For this review, take the finished solid that the model builds, in its own axes (mm). Face numbers are marked on the shaded views. A direction names the side the tool comes from. Give positions to 0.01 mm unless a question says otherwise; leave off trailing zeros. Loops run counter-clockwise (first coordinate to the right, second up) from the corner with the lowest first, then second, coordinate; pieces in that order, holes last. Notation, with made-up numbers: (-26, 33.5) -> (19, 33.5) arc R19 cw to (19, 70.5) -> close; hole circle Ø7 at (41.25, 26.25). An arc over 180 degrees is marked (long way). Answer as CSV lines item,"result". Start each with the question number.
Item 1: Add section A-A on y = -15.5. State the section outline as (x, z) points.
Item 2: Add section C-C on z = 7. State the section outline as (x, y) points.
Item 3: The part is to be moulded in two halves that separate along X. For the marked faces 4, 5 and 6, say which applies: +X half, -X half, draft (parallel to the pull), parting line (faces both ways), or undercut.
Item 4: For L1, parallel to Y at x = -15.5, z = 1.2; L2, parallel to Y at x = 17, z = 2.75, list the stretches that pass through material, from the lowest coordinate up. Write a range as from..to.
Item 5: Add section D-D on y = 0. State the section outline as (x, z) points, plus the area to 3 significant figures.
Item 6: Add section B-B on x = 0. State the section outline as (y, z) points, plus the area to 3 significant figures.
Item 7: Clearance check with flat-ended pins moving along their axes: P1, Ø6.5, axis at x = 16, y = 15, coming from the +Z side; P2, Ø4.5, axis at x = -17, z = 6, coming from the -Y side; P3, Ø4, axis at x = 16.5, z = 7.6, coming from the -Y side; P4, Ø23.5, axis at x = 0, y = 0, coming from the +Z side. State where each tip first meets the part, or that it passes through.
Item 8: Machinability: for the marked faces 1, 2 and 3, which of the approach directions +Z, -Z, +X, -X, +Y, -Y give a long, thin tool a straight path to every point of the face, cutting with its end or side? Answer none if there is none.
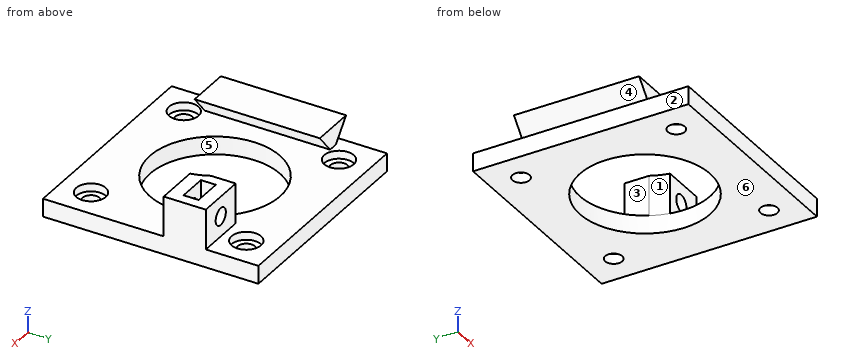
```python
from build123d import *

# Parameters (mm, degrees)
SKETCH_W        = 43
SKETCH_H        = 43
SKETCH_R        = 13
SKETCH_R_2      = 1.7
PAD_DEPTH       = 3.6
SKETCH001_R     = 2.95
POCKET_DEPTH    = 1.6
PAD001_DEPTH    = 8
SKETCH003_R     = 1.7
POCKET001_DEPTH = 18.901
POCKET002_DEPTH = 1.5
PAD002_DEPTH    = 12.5


with BuildPart() as part:
    # Sketch → Pad (new body)
    with BuildSketch(Plane.XY):
        Rectangle(SKETCH_W, SKETCH_H)
        Circle(SKETCH_R, mode=Mode.SUBTRACT)
        with Locations((-15.5, 15.5)):
            Circle(SKETCH_R_2, mode=Mode.SUBTRACT)
        with Locations((15.5, 15.5)):
            Circle(SKETCH_R_2, mode=Mode.SUBTRACT)
        with Locations((15.5, -15.5)):
            Circle(SKETCH_R_2, mode=Mode.SUBTRACT)
        with Locations((-15.5, -15.5)):
            Circle(SKETCH_R_2, mode=Mode.SUBTRACT)
    extrude(amount=PAD_DEPTH)

    # Sketch001 (on Face11 of Pad) → Pocket (cut)
    with BuildSketch(Plane.XY.offset(3.6)):
        with Locations((15.5, 15.5)):
            Circle(SKETCH001_R)
        with Locations((-15.5, 15.5)):
            Circle(SKETCH001_R)
        with Locations((-15.5, -15.5)):
            Circle(SKETCH001_R)
        with Locations((15.5, -15.5)):
            Circle(SKETCH001_R)
    extrude(amount=-POCKET_DEPTH, mode=Mode.SUBTRACT)

    # Sketch002 (on Face5 of Pocket) → Pad001 (join)
    with BuildSketch(Plane.XY.offset(3.6)):
        with BuildLine():
            ThreePointArc((12.737347, 2.6), (12.241687, 4.375053), (11.5, 6.062178))
            Line((11.5, 6.062178), (11.5, 11))
            Line((11.5, 11), (21.5, 11))
            Line((21.5, 11), (21.5, 2.6))
            Line((21.5, 2.6), (12.737347, 2.6))
        make_face()
    extrude(amount=PAD001_DEPTH)

    # Sketch003 (on Face10 of Pad001) → Pocket001 (cut, through all)
    with BuildSketch(Plane.XZ.offset(-2.6)):
        with Locations((16.5, 7.6)):
            Circle(SKETCH003_R)
    extrude(amount=-POCKET001_DEPTH, mode=Mode.SUBTRACT)

    # Sketch004 (on DatumPlane) → Pocket002 (cut, symmetric)
    with BuildSketch(Plane.XZ.offset(-6.8)):
        Polygon((13.598815, 5.925), (16.5, 4.25), (19.401185, 5.925), (19.401185, 15.925), (13.598815, 15.925), align=None)
    extrude(amount=POCKET002_DEPTH, both=True, mode=Mode.SUBTRACT)

    # Sketch005 → Pad002 (join, symmetric)
    with BuildSketch(Plane.XZ):
        Polygon((-22.9, 7.7), (-14.1, 7.7), (-18.5, 2.456284), align=None)
    extrude(amount=PAD002_DEPTH, both=True)


solid = part.part
```
Computed values:
1,outline,"(-21.5, 0) -> (-17.2, 0) -> (-17.2, 2) -> (-18.45, 2) -> (-18.45, 3.6) -> (-21.5, 3.6) -> close; (-13.8, 0) -> (13.8, 0) -> (13.8, 2) -> (12.55, 2) -> (12.55, 3.6) -> (-12.55, 3.6) -> (-12.55, 2) -> (-13.8, 2) -> close; (17.2, 0) -> (21.5, 0) -> (21.5, 3.6) -> (18.45, 3.6) -> (18.45, 2) -> (17.2, 2) -> close"
2,outline,"(-22.31, -12.5) -> (-14.69, -12.5) -> (-14.69, 12.5) -> (-22.31, 12.5) -> close; (11.5, 6.06) arc R13 cw to (12.74, 2.6) -> (14.91, 2.6) -> (14.91, 5.3) -> (13.6, 5.3) -> (13.6, 8.3) -> (14.91, 8.3) -> (14.91, 11) -> (11.5, 11) -> close; (18.09, 2.6) -> (21.5, 2.6) -> (21.5, 11) -> (18.09, 11) -> (18.09, 8.3) -> (19.4, 8.3) -> (19.4, 5.3) -> (18.09, 5.3) -> close"
3,face 4,"-X half"
3,face 5,"undercut"
3,face 6,"draft"
4,L1,"-21.5..-17.2, -13.8..13.8, 17.2..21.5"
4,L2,"-21.5..-18.04, -12.96..12.96, 18.04..21.5"
5,outline,"(-22.9, 7.7) -> (-19.46, 3.6) -> (-21.5, 3.6) -> (-21.5, 0) -> (-13, 0) -> (-13, 3.6) -> (-17.54, 3.6) -> (-14.1, 7.7) -> close; (13, 0) -> (21.5, 0) -> (21.5, 3.6) -> (13, 3.6) -> close"
5,area,"83.2 mm²"
6,outline,"(-21.5, 0) -> (-13, 0) -> (-13, 3.6) -> (-21.5, 3.6) -> close; (13, 0) -> (21.5, 0) -> (21.5, 3.6) -> (13, 3.6) -> close"
6,area,"61.2 mm²"
7,P1,"z = 3.6"
7,P2,"y = -12.5"
7,P3,"y = 2.6"
7,P4,"through"
8,face 1,"+Z, -Z, -Y"
8,face 2,"-Z, -X, +Y, -Y"
8,face 3,"+Z, +Y, -Y"
